from build123d import *

# Parameters (mm, degrees)
F0_R     = 2.1
F1_DEPTH = 960


with BuildPart() as f1:
    # F0 (on Front) → F1 (new body)
    with BuildSketch(Plane.XZ):
        with BuildLine():
            ThreePointArc((9.944745, 8.840758), (9.651851, 9.547865), (8.944745, 9.840758))
            Line((8.944745, 9.840758), (2.944745, 9.840758))
            Line((2.944745, 9.840758), (2.944745, 7.840758))
            Line((2.944745, 7.840758), (6.884085, 7.840758))
            Line((6.884085, 7.840758), (2.884085, 3.840758))
            Line((2.884085, 3.840758), (-2.994595, 3.840758))
            Line((-2.994595, 3.840758), (-6.994595, 7.840758))
            Line((-6.994595, 7.840758), (-3.055255, 7.840758))
            Line((-3.055255, 7.840758), (-3.055255, 9.840758))
            Line((-3.055255, 9.840758), (-9.055255, 9.840758))
            ThreePointArc((-9.055255, 9.840758), (-9.762362, 9.547865), (-10.055255, 8.840758))
            Line((-10.055255, 8.840758), (-10.055255, 2.840758))
            Line((-10.055255, 2.840758), (-8.055255, 2.840758))
            Line((-8.055255, 2.840758), (-8.055255, 6.780098))
            Line((-8.055255, 6.780098), (-4.055255, 2.780098))
            Line((-4.055255, 2.780098), (-4.055255, -3.098581))
            Line((-4.055255, -3.098581), (-8.055255, -7.098581))
            Line((-8.055255, -7.098581), (-8.055255, -3.159242))
            Line((-8.055255, -3.159242), (-10.055255, -3.159242))
            Line((-10.055255, -3.159242), (-10.055255, -10.159242))
            Line((-10.055255, -10.159242), (-10.055255, -17.159242))
            Line((-10.055255, -17.159242), (-8.055255, -17.159242))
            Line((-8.055255, -17.159242), (-8.055255, -13.219902))
            Line((-8.055255, -13.219902), (-4.055255, -17.219902))
            Line((-4.055255, -17.219902), (-4.055255, -23.098581))
            Line((-4.055255, -23.098581), (-8.055255, -27.098581))
            Line((-8.055255, -27.098581), (-8.055255, -23.159242))
            Line((-8.055255, -23.159242), (-10.055255, -23.159242))
            Line((-10.055255, -23.159242), (-10.055255, -29.159242))
            ThreePointArc((-10.055255, -29.159242), (-9.762362, -29.866348), (-9.055255, -30.159242))
            Line((-9.055255, -30.159242), (-3.055255, -30.159242))
            Line((-3.055255, -30.159242), (-3.055255, -28.159242))
            Line((-3.055255, -28.159242), (-6.994595, -28.159242))
            Line((-6.994595, -28.159242), (-2.994595, -24.159242))
            Line((-2.994595, -24.159242), (2.884085, -24.159242))
            Line((2.884085, -24.159242), (6.884085, -28.159242))
            Line((6.884085, -28.159242), (2.944745, -28.159242))
            Line((2.944745, -28.159242), (2.944745, -30.159242))
            Line((2.944745, -30.159242), (8.944745, -30.159242))
            ThreePointArc((8.944745, -30.159242), (9.651851, -29.866348), (9.944745, -29.159242))
            Line((9.944745, -29.159242), (9.944745, -23.159242))
            Line((9.944745, -23.159242), (7.944745, -23.159242))
            Line((7.944745, -23.159242), (7.944745, -27.098581))
            Line((7.944745, -27.098581), (3.944745, -23.098581))
            Line((3.944745, -23.098581), (3.944745, -17.219902))
            Line((3.944745, -17.219902), (7.944745, -13.219902))
            Line((7.944745, -13.219902), (7.944745, -17.159242))
            Line((7.944745, -17.159242), (9.944745, -17.159242))
            Line((9.944745, -17.159242), (9.944745, -10.159242))
            Line((9.944745, -10.159242), (9.944745, -3.159242))
            Line((9.944745, -3.159242), (7.944745, -3.159242))
            Line((7.944745, -3.159242), (7.944745, -7.098581))
            Line((7.944745, -7.098581), (3.944745, -3.098581))
            Line((3.944745, -3.098581), (3.944745, 2.780098))
            Line((3.944745, 2.780098), (7.944745, 6.780098))
            Line((7.944745, 6.780098), (7.944745, 2.840758))
            Line((7.944745, 2.840758), (9.944745, 2.840758))
            Line((9.944745, 2.840758), (9.944745, 8.840758))
        make_face()
        with Locations((-0.055255, -20.159242)):
            Circle(F0_R, mode=Mode.SUBTRACT)
        Polygon((-2.994595, -4.159242), (2.884085, -4.159242), (7.944745, -9.219902), (7.944745, -10.159242), (7.944745, -11.098581), (2.884085, -16.159242), (-2.994595, -16.159242), (-8.055255, -11.098581), (-8.055255, -10.159242), (-8.055255, -9.219902), align=None, mode=Mode.SUBTRACT)
        with Locations((-0.055255, -0.159242)):
            Circle(F0_R, mode=Mode.SUBTRACT)
    extrude(amount=F1_DEPTH)


solid = f1.part
Could you check a few things on this model? Use its own coordinates, in mm. Give positions to 0.01 mm unless a question says otherwise; leave off trailing zeros. Return JSON: item names as keys, results as strings.
Item 1: I'm going to push flat-ended pins straight in: pin 1 (3 mm diameter, centred on y = -458.5, z = 0, fed in from -X); pin 2 (1 mm diameter, centred on x = -7.5, z = -3.5, fed in from +Y). Where does each tip first touch, or does it pass through?
Geometry results:
{"pin 1": "stops at x = -4.06", "pin 2": "passes through"}
Item 2: I need wall thicknesses on L1, parallel to Z at x = 8, y = -679; L2, parallel to Z at x = 0, y = -838; L3, parallel to Z at x = -8, y = -530. Which ranges of each line are inside material? Lowest first, please. Write a range as from..to.
Geometry results:
{"L1": "z = -30.16..-23.16, -17.16..-3.16, 2.84..9.84", "L2": "z = -24.16..-22.26, -18.06..-16.16, -4.16..-2.26, 1.94..3.84", "L3": "z = -30.16..-27.04, -13.28..-11.15, -9.16..-7.04, 6.72..9.84"}
Item 3: If we section it at A-A on y = -704: Count the separate pieces of the cut face and the enclosed holes in it, plus the area to 3 significant figures.
Geometry results:
{"separate pieces": "1", "enclosed holes": "3", "area": "322 mm²"}
